Source: CAD feature listing. Evaluate the final solid. Frame: model axes, mm. Face numbers are marked on the shaded views. A direction names the side the tool comes from. Give positions to 0.01 mm unless a question says otherwise; leave off trailing zeros. Write each loop counter-clockwise with the first axis right and the second up, starting at its lowest first coordinate (ties: lowest second). Pieces come first, ordered by that corner, then holes. Notation, with made-up numbers: (87, 23) - (114, 23) arc R18 cw to (114, 51) - close; hole circle Ø4 at (57, -13). An arc over 180 degrees is marked (long way). Answer as a JSON object with one key per item and string values. Group by question number.
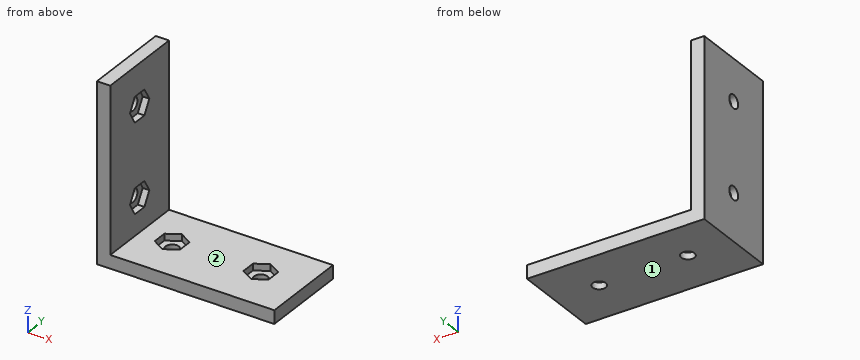
from build123d import *

# Parameters (mm, degrees)
ESQUISSE1_W             = 40
ESQUISSE1_H             = 20
BOSS_EXTRU_1_DEPTH      = 3
ESQUISSE2_R             = 1.5
ENL_V_MAT_EXTRU_1_DEPTH = 3
ESQUISSE3_W             = 3
ESQUISSE3_H             = 20
BOSS_EXTRU_2_DEPTH      = 37
ESQUISSE4_R             = 1.5
ENL_V_MAT_EXTRU_2_DEPTH = 3
ENL_V_MAT_EXTRU_3_DEPTH = 1.5
ENL_V_MAT_EXTRU_4_DEPTH = 1.5


with BuildPart() as part:
    # Esquisse1 → Boss.-Extru.1 (new body)
    with BuildSketch(Plane.XY):
        with Locations((20, 10)):
            Rectangle(ESQUISSE1_W, ESQUISSE1_H)
    extrude(amount=BOSS_EXTRU_1_DEPTH)

    # Esquisse2 → Enlèv. mat.-Extru.1 (cut)
    with BuildSketch(Plane.XY.offset(3)):
        with Locations((10, 10.5)):
            Circle(ESQUISSE2_R)
        with Locations((30, 10.5)):
            Circle(ESQUISSE2_R)
    extrude(amount=-ENL_V_MAT_EXTRU_1_DEPTH, mode=Mode.SUBTRACT)

    # Esquisse3 → Boss.-Extru.2 (add)
    with BuildSketch(Plane.XY.offset(3)):
        with Locations((1.5, 10)):
            Rectangle(ESQUISSE3_W, ESQUISSE3_H)
    extrude(amount=BOSS_EXTRU_2_DEPTH)

    # Esquisse4 → Enlèv. mat.-Extru.2 (cut)
    with BuildSketch(Plane.ZY):
        with Locations((10.6, 10)):
            Circle(ESQUISSE4_R)
        with Locations((30.6, 10)):
            Circle(ESQUISSE4_R)
    extrude(amount=-ENL_V_MAT_EXTRU_2_DEPTH, mode=Mode.SUBTRACT)

    # Esquisse5 → Enlèv. mat.-Extru.3 (cut)
    with BuildSketch(Plane(origin=(3, 0, 0), x_dir=(0, 0, -1), z_dir=(1, 0, 0))):
        Polygon((-13.45, 8.354551733), (-10.6, 6.709103466), (-7.75, 8.354551733), (-7.75, 11.645448267), (-10.6, 13.290896534), (-13.45, 11.645448267), align=None)
        Polygon((-30.6, 6.709103466), (-27.75, 8.354551733), (-27.75, 11.645448267), (-30.6, 13.290896534), (-33.45, 11.645448267), (-33.45, 8.354551733), align=None)
    extrude(amount=-ENL_V_MAT_EXTRU_3_DEPTH, mode=Mode.SUBTRACT)

    # Esquisse6 → Enlèv. mat.-Extru.4 (cut)
    with BuildSketch(Plane.XY.offset(3)):
        Polygon((27.15, 8.854551733), (30, 7.209103466), (32.85, 8.854551733), (32.85, 12.145448267), (30, 13.790896534), (27.15, 12.145448267), align=None)
        Polygon((10, 7.209103466), (12.85, 8.854551733), (12.85, 12.145448267), (10, 13.790896534), (7.15, 12.145448267), (7.15, 8.854551733), align=None)
    extrude(amount=-ENL_V_MAT_EXTRU_4_DEPTH, mode=Mode.SUBTRACT)


solid = part.part
Q1. Section A-A on x = 30.5. Return the cut outline in (y, z).
Q2. Ray query, probe 1 along Z at (x, y) = (23.5, 10.25). Return the intervals inside material, ascending. Write a range as [from, to].
Q3. Reachability of the marked faces 1 and 2 from +Z, -Z, +X, -X, +Y, -Y: full face, straight path, thin tool, end or side. Return the list, or none.
Q4. First-contact query: pin 1 Ø3 at (y, z) = (8.5, 30) entering from +X; pin 2 Ø1.5 at (x, z) = (7, 5.5) entering from +Y; pin 3 Ø5 at (x, y) = (25, 8.5) entering from +Z; pin 4 Ø1.7 at (x, y) = (30.5, 12) entering from +Z. Flat tips, straight axial feed; report the tip coordinate or a pass-through.
Q5. Section C-C on x = 4.5. Return the cut outline in (y, z).
Q6. Section B-B on y = 5.25. Return the cut outline in (x, z), then the cut area to 3 significant figures.
Q7. Section D-D on z = 23. Return the cut outline in (x, y).
Taken from the geometry:
{
 "1": {"outline": "(0, 0) - (9.09, 0) - (9.09, 1.5) - (7.5, 1.5) - (7.5, 3) - (0, 3) - close; (11.91, 0) - (20, 0) - (20, 3) - (13.5, 3) - (13.5, 1.5) - (11.91, 1.5) - close"},
 "2": {"probe 1": "z = [0, 3]"},
 "3": {"face 1": "-Z, +X, -X, +Y, -Y", "face 2": "+Z, +X, +Y, -Y"},
 "4": {"pin 1": "stops at x = 3", "pin 2": "passes through", "pin 3": "stops at z = 3", "pin 4": "stops at z = 1.5"},
 "5": {"outline": "(0, 0) - (20, 0) - (20, 3) - (0, 3) - close"},
 "6": {"outline": "(0, 0) - (40, 0) - (40, 3) - (3, 3) - (3, 40) - (0, 40) - close", "area": "231 mm²"},
 "7": {"outline": "(0, 0) - (3, 0) - (3, 20) - (0, 20) - close"}
}
